```python
from build123d import *
from build123d.topology import SkipClean

# Parameters (mm, degrees)
SKETCH1_R           = 26.15
SKETCH1_R_2         = 20.4
BOSS_EXTRUDE1_DEPTH = 30
BOSS_EXTRUDE7_DEPTH = 10
SKETCH11_R          = 26
SKETCH11_R_2        = 18
EXTRUDE_THIN1_DEPTH = 145
BOSS_EXTRUDE8_START = 10
BOSS_EXTRUDE8_DEPTH = 10


with BuildPart() as part:
    # Sketch1 → Boss-Extrude1 (new body)
    with BuildSketch(Plane.XY):
        Circle(SKETCH1_R)
        Circle(SKETCH1_R_2, mode=Mode.SUBTRACT)
    extrude(amount=BOSS_EXTRUDE1_DEPTH)

    # Sketch10 → Boss-Extrude7 (add)
    with BuildSketch(Plane.XY.offset(30)):
        with BuildLine():
            Line((-26, 65), (-26, 0))
            ThreePointArc((-26, 0), (0, -26), (26, 0))
            Line((26, 0), (26, 65))
            ThreePointArc((26, 65), (0, 91), (-26, 65))
        make_face()
    extrude(amount=-BOSS_EXTRUDE7_DEPTH)

    # Sketch11 → Extrude-Thin1 (add)
    with SkipClean():  # the faces are left unmerged after this step: merging them gives an invalid solid
        with BuildSketch(Plane(origin=(0, 0, 20), x_dir=(-1, 0, 0), z_dir=(0, 0, -1))):
            with Locations((0, 65)):
                Circle(SKETCH11_R)
            with Locations((0, 65)):
                Circle(SKETCH11_R_2, mode=Mode.SUBTRACT)
        extrude(amount=EXTRUDE_THIN1_DEPTH)
    add(part.part.scale(1), mode=Mode.REPLACE)  # the faces are merged on a copy

    # Sketch12 → Boss-Extrude8 (add)
    with SkipClean():  # the faces are left unmerged after this step: merging them gives an invalid solid
        with BuildSketch(Plane(origin=(0, 0, -125), x_dir=(-1, 0, 0), z_dir=(0, 0, -1)).offset(BOSS_EXTRUDE8_START)):
            with BuildLine():
                ThreePointArc((26.002446969, 63.939646719), (0.305760086, 91.449477206), (-26.613467545, 65.134734686))
                Line((-26.613467545, 65.134734686), (-26.610802329, 64.76017088))
                Line((-26.610802329, 64.76017088), (-26.15, 0))
                ThreePointArc((-26.15, 0), (0, -26.15), (26.15, 0))
                Line((26.15, 0), (26.149721481, 0.120691665))
                Line((26.149721481, 0.120691665), (26.002446969, 63.939646719))
            make_face()
        extrude(amount=-BOSS_EXTRUDE8_DEPTH)


solid = part.part
```
CAD build for the part. Positions are in the model's coordinates, mm. A direction names the side the tool comes from. Round coordinates to 2 decimals unless told otherwise and drop trailing zeros. Order: outer loops, then holes, each group sorted by start corner. A loop starts at its lowest first (then second) coordinate and runs counter-clockwise, first axis right, second up.
Q1. Two-plate mould, pull along Y, no slides. Class faces 1 (the flat face through (1, 7, -125)), 2 (the cylindrical face through (0.575, -26.144, -130.07)), 3 (the flat face through (0, 65, 20)): pulls with the +Y half, pulls with the -Y half, needs draft (parallel to the pull), parting line crosses it, or undercut.
Q2. Wall check: L1, parallel to Y at x = 0, z = 5.25; L2, parallel to Z at x = -19.5, y = 31; L3, parallel to Y at x = 0, z = -71. Give the ranges that are in metal, low to high.
Q3. Drop flat-ended pins along their axis: pin 1 (1 mm diameter, centred on x = 11.5, z = -17.5, fed in from -Y); pin 2 (6 mm diameter, centred on y = 62, z = 5, fed in from -X); pin 3 (8 mm diameter, centred on x = 13, z = -26.5, fed in from +Y). Give the stop position or say it passes through.
Q4. Which spindle directions (+Z, -Z, +X, -X, +Y, -Y) get a long thin tool onto all of the face, cutting with end or side? Do faces 4 (the flat face through (0, 33, 30)), 5 (the cylindrical face through (2.343, 82.847, -51.485)), 6 (the flat face through (-26, 34, 25)), 7 (the flat face through (-13.7, -15.4, 0)), 8 (the flat face through (26, 33, 25)). Say none if no direction does.
Q5. Slice it at C-C (y = 76.5). Write the cut outline in (x, z).
Q6. Slice it at A-A (y = 36.5). Write the cut outline in (x, z), and give its area (3 significant figures).
Q7. Slice it at D-D (x = 0). Write the cut outline in (y, z).
Q8. Slice it at B-B (z = -46.5). Write the cut outline in (x, y), and give its area (3 significant figures).
Results below:
1. face 1: needs draft
1. face 2: pulls with the -Y half
1. face 3: undercut
2. L1: y = -26.15 to -20.4, 20.4 to 26.15, 39 to 47, 83 to 91
2. L2: z = -135 to -125, 20 to 30
2. L3: y = 39 to 47, 83 to 91
3. pin 1: stops at y = 41.44
3. pin 2: stops at x = -26
3. pin 3: stops at y = 89.39
4. face 4: +Z, +X, -X, +Y, -Y
4. face 5: none
4. face 6: +Z, -X, +Y
4. face 7: +X, -X, -Y
4. face 8: +Z, +X, +Y
5. outline: (-23.45, -135) - (24.03, -135) - (24.03, -125) - (23.32, -125) - (23.32, 30) - (-23.32, 30) - (-23.32, -125) - (-23.45, -125) - close; hole (-13.85, -125) - (13.85, -125) - (13.85, 20) - (-13.85, 20) - close
6. outline: (-26.07, -135) - (26.41, -135) - (26.41, -125) - (-26.07, -125) - close; (-26, 20) - (26, 20) - (26, 30) - (-26, 30) - close
6. area: 1,040 mm2
7. outline: (-26.15, -135) - (91.45, -135) - (91.45, -125) - (91, -125) - (91, 30) - (-26.15, 30) - (-26.15, 0) - (-20.4, 0) - (-20.4, 20) - (20.4, 20) - (20.4, 0) - (26.15, 0) - (26.15, 20) - (39, 20) - (39, -125) - (-26.15, -125) - close; hole (47, -125) - (83, -125) - (83, 20) - (47, 20) - close
8. outline: circle Ø52 at (0, 65); hole circle Ø36 at (0, 65)
8. area: 1,110 mm2
